Answer from the drawing. Dimensions are ordinates in mm from the lowest x, y and z of the part. A direction names the side the tool comes from. Give positions to 0.01 mm unless a question says otherwise; leave off trailing zeros. Order: outer loops, then holes, each group sorted by start corner. A loop starts at its lowest first (then second) coordinate and runs counter-clockwise, first axis right, second up. Notation, with made-up numbers: (9.5, 31) - (29.5, 31) arc R27 ccw to (29.5, 68) - close; hole circle Ø5 at (59, 22). An arc over 180 degrees is marked (long way). Use a Markdown table: item, result. Add a question column.
1) Find section B-B, the plane x = 300. Determine the outline of the cut face in (y, z).
2) For the marked faces 1, 2 and 3, determine the directions among +Z, -Z, +X, -X, +Y, -Y from which every point of the face is accessible in a straight line to the end or side of a thin tool.
3) Flat-ended cylindrical pins translate along their axes: pin 1 (12 mm diameter, centred on x = 144, z = 37.5, fed in from +Y); pin 2 (5 mm diameter, centred on x = 171, z = 66, fed in from -Y); pin 3 (12 mm diameter, centred on y = 216.5, z = 14, fed in from +X); pin 4 (24 mm diameter, centred on y = 22.5, z = 35.5, fed in from -X). Find the tip coordinate at first contact, or state that the pin passes through.
4) Find section A-A, the plane z = 47. Determine the outline of the cut face in (x, y), plus the area to 3 significant figures.
5) Straight lines are drawn through the part: line 1 (Y direction, x = 510, z = 113); line 2 (Y direction, x = 299, z = 7); line 3 (Y direction, x = 90, z = 116). For each, find the intervals that lie inside material, in ascending order.
6) The mould has two halves that part along X. Classify the marked faces 4, 5 and 6: released by +X, released by -X, zero draft, split by the parting line, or undercut.
7) Find section D-D, the plane y = 57. Determine the outline of the cut face in (x, z), plus the area to 3 significant figures.
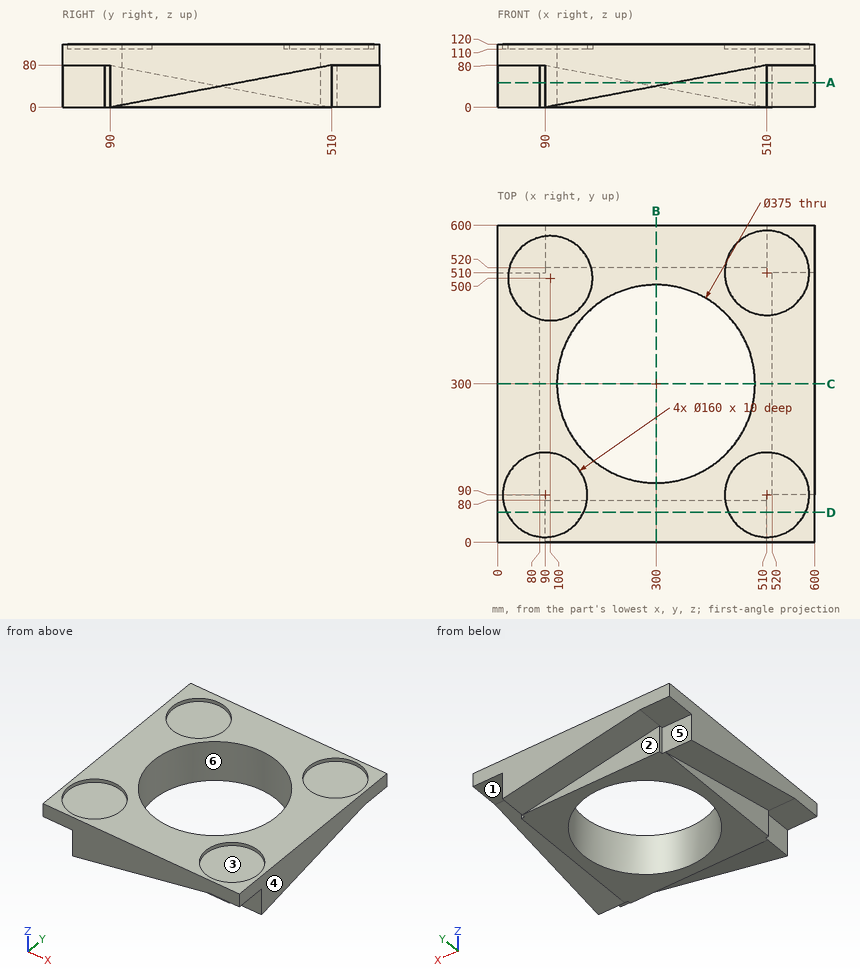
The answers:
| question | item | result |
|---|---|---|
| 1 | outline | (0, 40) - (80, 40) - (80, 0) - (112.5, 0) - (112.5, 120) - (0, 120) - close; (487.5, 0) - (520, 0) - (520, 40) - (600, 40) - (600, 120) - (487.5, 120) - close |
| 2 | face 1 | -Z, +X, +Y |
| 2 | face 2 | -Z, -X, +Y |
| 2 | face 3 | +Z |
| 3 | pin 1 | y = 520 |
| 3 | pin 2 | y = 0 |
| 3 | pin 3 | x = 520 |
| 3 | pin 4 | x = 90 |
| 4 | outline | (0, 263.25) - (80, 263.25) - (80, 90) - (90, 90) - (90, 0) - (336.75, 0) - (336.75, 80) - (510, 80) - (510, 90) - (600, 90) - (600, 336.75) - (520, 336.75) - (520, 510) - (510, 510) - (510, 600) - (263.25, 600) - (263.25, 520) - (90, 520) - (90, 510) - (0, 510) - close; hole circle Ø375 at (300, 300) |
| 4 | area | 162,000 mm2 |
| 5 | line 1 | 0 to 10, 170 to 430, 590 to 600 |
| 5 | line 2 | 80 to 112.5, 487.5 to 520 |
| 5 | line 3 | 0 to 10, 170 to 420.63, 579.37 to 600 |
| 6 | face 4 | released by +X |
| 6 | face 5 | zero draft |
| 6 | face 6 | undercut |
| 7 | outline | (0, 80) - (90, 80) - (90, 0) - (510, 80) - (600, 80) - (600, 120) - (582.88, 120) - (582.88, 110) - (437.12, 110) - (437.12, 120) - (162.88, 120) - (162.88, 110) - (17.12, 110) - (17.12, 120) - (0, 120) - close |
| 7 | area | 37,900 mm2 |
